Autodesk Inventor part; units mm, degrees
ref_plane "Work Plane1" through (54.5, 0, 0) normal (-1, 0, 0) x (0, 0, 1)
ref_plane "Work Plane2" through (0, 0, 7.25) normal (0, 0, 1) x (1, 0, 0)
ref_plane "YZ Plane" through (0, 0, 0) normal (1, 0, 0) x (0, 1, 0)
sketch "Sketch1" plane through (0, 0, 0) normal (0, 0, 1) x (1, 0, 0)
  line L0 (0, 0) -> (83.5, 0)
  line L1 (83.5, 0) -> (83.5, 70)
  line L2 (83.5, 70) -> (0, 70)
  line L3 (0, 70) -> (0, 0)
  dimension "d0" = 70
  dimension "d1" = 83.5
extrude "Extrusion1" add sketch "Sketch1" along normal blind 2
sketch "Sketch2" plane through (0, 0, 2) normal (0, 0, 1) x (1, 0, 0)
  line L0 (0, 70) -> (0, 0)
  line L1 (0, 35) -> (83.5, 35) construction
  line L2 (83.5, 0) -> (83.5, 70)
  line L3 (6.95, 31.4) -> (-5, 31.4) construction
  line L4 (-5, 31.4) -> (-5, 38.6) construction
  line L5 (-5, 38.6) -> (6.95, 38.6) construction
  line L6 (6.95, 38.6) -> (6.95, 31.4) construction
  line L7 (6.95, 31.4) -> (-5, 38.6) construction
  line L8 (-5, 31.4) -> (6.95, 38.6) construction
  line L9 (49.5, 34.65) -> (49.5, 29.45) construction
  line L10 (6.95, 31.4) -> (4.95, 31.4)
  line L11 (4.95, 31.4) -> (4.95, 21.85)
  line L12 (4.95, 21.85) -> (6.95, 21.85)
  line L13 (6.95, 21.85) -> (6.95, 31.4)
  line L14 (6.95, 38.6) -> (4.95, 38.6)
  line L15 (4.95, 38.6) -> (4.95, 45.2)
  line L16 (4.95, 45.2) -> (6.95, 45.2)
  line L17 (6.95, 45.2) -> (6.95, 38.6)
  line L18 (6.95, 45.2) -> (37.55, 45.2)
  line L19 (37.55, 45.2) -> (37.55, 43.2)
  line L20 (37.55, 43.2) -> (6.95, 43.2)
  line L21 (6.95, 43.2) -> (6.95, 45.2)
  line L22 (37.55, 45.2) -> (39.55, 45.2)
  line L23 (39.55, 45.2) -> (39.55, 38.6)
  line L24 (39.55, 38.6) -> (37.55, 38.6)
  line L25 (37.55, 38.6) -> (37.55, 45.2)
  line L26 (37.55, 31.4) -> (39.55, 31.4)
  line L27 (39.55, 31.4) -> (39.55, 21.85)
  line L28 (39.55, 21.85) -> (37.55, 21.85)
  line L29 (37.55, 21.85) -> (37.55, 31.4)
  line L30 (6.95, 21.85) -> (37.55, 21.85)
  line L31 (37.55, 21.85) -> (37.55, 11.6)
  line L32 (37.55, 11.6) -> (6.95, 11.6)
  line L33 (6.95, 11.6) -> (6.95, 21.85)
  point P0 (0.975, 35)
  dimension "d8" = 7.2
  dimension "d13" = 11.95
  dimension "d14" = 5
  dimension "d19" = 2
  dimension "d20" = 23.4
  dimension "d21" = 10.25
  dimension "d22" = 30.6
  dimension "d23" = 2
  dimension "d24" = 2
  dimension "d25" = 33.6
  dimension "d30" = 11.95
extrude "Extrusion2" add sketch "Sketch2" along normal blind 4 contours L13 L12 L11 L10 | L29 L26 L27 L28 | L14 L15 L16 L17 | L17 L18 L19 L20 | L19 L22 L23 L24 L25
extrude "Extrusion3" cut sketch "Sketch2" against normal blind 2 contours L30 L31 L32 L33
ref_plane "Work Plane1" through (54.5, 0, 0) normal (-1, 0, 0) x (0, 0, 1)
sketch "Sketch3" plane through (54.5, 0, 0) normal (-1, 0, 0) x (0, 0, 1)
  arc A0 (7.25, 30.5) -> (7.25, 39.5) centre (7.25, 35) ccw
  circle A1 centre (7.25, 35) radius 3.5
  line L0 (2, 21.85) -> (2, 31.4)
  line L1 (7.25, 39.5) -> (2, 39.5)
  line L2 (2, 39.5) -> (2, 30.5)
  line L3 (2, 30.5) -> (7.25, 30.5)
  line L4 (7.25, 30.5) -> (7.25, 39.5) construction
  arc A2 (7.25, 39.5) -> (7.25, 30.5) centre (7.25, 35) ccw construction
  line L5 (2, 38.6) -> (6, 38.6)
  line L6 (2, 31.4) -> (6, 31.4)
  line L7 (6, 38.6) -> (6, 31.4) construction
  line L8 (6, 35) -> (7.25, 35) construction
  point P0 (0, 0)
  dimension "d32" = 9
  dimension "d33" = 7
  dimension "d34" = 5.25
ref_plane "Work Plane2" through (0, 0, 7.25) normal (0, 0, 1) x (1, 0, 0)
sketch "Sketch4" plane through (0, 0, 7.25) normal (0, 0, 1) x (1, 0, 0)
  line L0 (39.55, 38.6) -> (37.55, 38.6)
  line L1 (37.55, 31.4) -> (39.55, 31.4)
  line L2 (39.55, 38.6) -> (39.55, 31.4) construction
  line L3 (39.55, 35) -> (54.5, 35) construction
  line L4 (54.5, 35) -> (59.5, 35)
  point P0 (0, 0)
  dimension "d36" = 14.95
  dimension "d37" = 5
sweep "Sweep1" add profiles "Sketch3" path "Sketch4" path curves L4
sketch "Sketch7" plane through (0, 0, 2) normal (0, 0, 1) x (1, 0, 0)
  line L0 (40, 65) -> (78.5, 65) construction
  line L1 (78.5, 65) -> (78.5, 5) construction
  line L2 (78.5, 5) -> (40, 5) construction
  line L3 (40, 5) -> (40, 65) construction
  line L4 (83.5, 70) -> (0, 70)
  line L5 (0, 70) -> (0, 0)
  line L6 (83.5, 0) -> (83.5, 70)
  line L7 (0, 0) -> (83.5, 0)
  circle A0 centre (40, 65) radius 1.6
  circle A1 centre (78.5, 65) radius 1.6
  circle A2 centre (40, 5) radius 1.6
  circle A3 centre (78.5, 5) radius 1.6
  dimension "d54" = 5
  dimension "d55" = 40
  dimension "d56" = 5
  dimension "d57" = 5
  dimension "d58" = 3.2
  dimension "d59" = 3.2
  dimension "d60" = 3.2
  dimension "d61" = 3.2
extrude "Extrusion6" cut sketch "Sketch7" against normal blind 5 contours A0 | A1 | A2 | A3
sketch "Sketch8" plane through (0, 0, 2) normal (0, 0, 1) x (1, 0, 0)
  circle A0 centre (40, 65) radius 1.6
  line L0 (40, 68.4641) -> (43, 66.7321)
  line L1 (43, 66.7321) -> (43, 63.2679)
  line L2 (43, 63.2679) -> (40, 61.5359)
  line L3 (40, 61.5359) -> (37, 63.2679)
  line L4 (37, 63.2679) -> (37, 66.7321)
  line L5 (37, 66.7321) -> (40, 68.4641)
  line L6 (40, 69.6188) -> (44, 67.3094)
  line L7 (44, 67.3094) -> (44, 62.6906)
  line L8 (44, 62.6906) -> (40, 60.3812)
  line L9 (40, 60.3812) -> (36, 62.6906)
  line L10 (36, 62.6906) -> (36, 67.3094)
  line L11 (36, 67.3094) -> (40, 69.6188)
  circle A1 centre (78.5, 5) radius 1.6
  line L12 (40, 65) -> (78.5, 65) construction
  line L13 (78.5, 65) -> (78.5, 5) construction
  line L14 (78.5, 5) -> (40, 5) construction
  line L15 (40, 5) -> (40, 65) construction
  line L16 (78.5, 61.5359) -> (75.5, 63.2679)
  line L17 (75.5, 63.2679) -> (75.5, 66.7321)
  line L18 (75.5, 66.7321) -> (78.5, 68.4641)
  line L19 (78.5, 68.4641) -> (81.5, 66.7321)
  line L20 (81.5, 66.7321) -> (81.5, 63.2679)
  line L21 (81.5, 63.2679) -> (78.5, 61.5359)
  line L22 (78.5, 60.3812) -> (74.5, 62.6906)
  line L23 (74.5, 62.6906) -> (74.5, 67.3094)
  line L24 (74.5, 67.3094) -> (78.5, 69.6188)
  line L25 (78.5, 69.6188) -> (82.5, 67.3094)
  line L26 (82.5, 67.3094) -> (82.5, 62.6906)
  line L27 (82.5, 62.6906) -> (78.5, 60.3812)
  line L28 (78.5, 8.4641) -> (81.5, 6.7321)
  line L29 (81.5, 6.7321) -> (81.5, 3.2679)
  line L30 (81.5, 3.2679) -> (78.5, 1.5359)
  line L31 (78.5, 1.5359) -> (75.5, 3.2679)
  line L32 (75.5, 3.2679) -> (75.5, 6.7321)
  line L33 (75.5, 6.7321) -> (78.5, 8.4641)
  line L34 (78.5, 9.6188) -> (82.5, 7.3094)
  line L35 (82.5, 7.3094) -> (82.5, 2.6906)
  line L36 (82.5, 2.6906) -> (78.5, 0.3812)
  line L37 (78.5, 0.3812) -> (74.5, 2.6906)
  line L38 (74.5, 2.6906) -> (74.5, 7.3094)
  line L39 (74.5, 7.3094) -> (78.5, 9.6188)
  line L40 (40, 9.6188) -> (44, 7.3094)
  line L41 (44, 7.3094) -> (44, 2.6906)
  line L42 (44, 2.6906) -> (40, 0.3812)
  line L43 (40, 0.3812) -> (36, 2.6906)
  line L44 (36, 2.6906) -> (36, 7.3094)
  line L45 (36, 7.3094) -> (40, 9.6188)
  line L46 (40, 8.4641) -> (43, 6.7321)
  line L47 (43, 6.7321) -> (43, 3.2679)
  line L48 (43, 3.2679) -> (40, 1.5359)
  line L49 (40, 1.5359) -> (37, 3.2679)
  line L50 (37, 3.2679) -> (37, 6.7321)
  line L51 (37, 6.7321) -> (40, 8.4641)
  point P0 (0, 0)
  dimension "d64" = 6
  dimension "d65" = 1
  dimension "d66" = 6
  dimension "d67" = 1
  dimension "d68" = 6
  dimension "d69" = 1
  dimension "d70" = 1
  dimension "d71" = 6
sketch "Sketch6" plane through (0, 70, 0) normal (0, 1, 0) x (1, 0, 0)
  line L0 (83.5, -2) -> (0, -2)
  line L1 (79, -2) -> (79, -7.25)
  arc A0 (70, -7.25) -> (79, -7.25) centre (74.5, -7.25) ccw
  line L2 (70, -7.25) -> (70, -2)
  circle A1 centre (74.5, -7.25) radius 3.5
  line L3 (39.55, -2) -> (39.55, -6)
  point P0 (0, 0)
  dimension "d48" = 7
  dimension "d49" = 4.5
  dimension "d50" = 5.25
  dimension "d51" = 34.95
properties part number "middleBase"
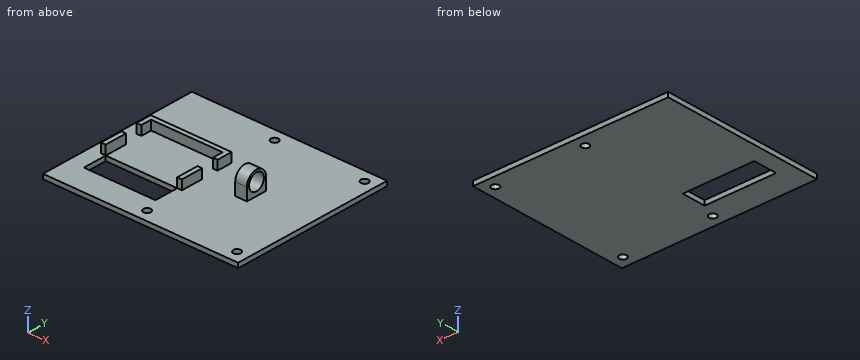
CAD build for the part. Positions are in the model's coordinates, mm. Give positions to 0.01 mm unless a question says otherwise; leave off trailing zeros. Loops run counter-clockwise (first coordinate to the right, second up) from the corner with the lowest first, then second, coordinate; pieces in that order, holes last. Notation, with made-up numbers: M -28.5,-3.75 L 1.5,-3.75 A21 cw 1.5,8.25 Z; hole C 25,66 d10. An arc over 180 degrees is marked long. Answer in a Markdown table with one row per item. Add a question column.
Item 1: Band-saw the part on C-C on x = 78.5. Give the cut face in (y, z).
Item 2: Probe probe 1 along X at (y, z) = (65, 1); probe 2 along Y at (x, z) = (40, 0.4); probe 3 along Z at (x, y) = (15.5, 11). List the from-to ranges inside material, lowest first.
Item 3: Band-saw the part on B-B on x = 35. Give the cut face in (y, z).
Item 4: Band-saw the part on D-D on y = 35. Give the cut face in (x, z).
Item 5: Drop flat-ended pins along their axis: P1, Ø2, axis at x = 29.5, z = 5, coming from the -Y side; P2, Ø3, axis at x = 40, y = 5, coming from the +Z side; P3, Ø2, axis at y = 26, z = 5, coming from the -X side; P4, Ø2.5, axis at x = 56.5, z = 4.5, coming from the -Y side. Give the stop position or say it passes through.
Item 6: Band-saw the part on A-A on y = 5. Give the cut face in (x, z), then the cut area to 3 significant figures.
Reply:
| question | item | result |
|---|---|---|
| 1 | outline | M 0,0 L 3.4,0 L 3.4,2 L 0,2 Z; M 6.6,0 L 63.4,0 L 63.4,2 L 6.6,2 Z; M 66.6,0 L 70,0 L 70,2 L 66.6,2 Z |
| 2 | probe 1 | x = 0 to 38.4, 41.6 to 76.9, 80.1 to 83.5 |
| 2 | probe 2 | y = 0 to 3.4, 6.6 to 63.4, 66.6 to 70 |
| 2 | probe 3 | z = 0 to 2 |
| 3 | outline | M 0,0 L 11.6,0 L 11.6,2 L 0,2 Z; M 21.85,0 L 70,0 L 70,2 L 45.2,2 L 45.2,6 L 43.2,6 L 43.2,2 L 21.85,2 Z |
| 4 | outline | M 0,0 L 83.5,0 L 83.5,2 L 59.5,2 L 59.5,3.75 L 54.5,3.75 L 54.5,2 L 0,2 Z; M 54.5,10.75 L 59.5,10.75 L 59.5,11.75 L 54.5,11.75 Z |
| 5 | P1 | stops at y = 43.2 |
| 5 | P2 | passes through |
| 5 | P3 | stops at x = 4.95 |
| 5 | P4 | stops at y = 30.5 |
| 6 | outline | M 0,0 L 38.4,0 L 38.4,2 L 0,2 Z; M 41.6,0 L 76.9,0 L 76.9,2 L 41.6,2 Z; M 80.1,0 L 83.5,0 L 83.5,2 L 80.1,2 Z |
| 6 | area | 154 mm^2 |
